For this review, take the finished solid that the model builds, in its own axes (mm). Give positions to 0.01 mm unless a question says otherwise; leave off trailing zeros. Write each loop counter-clockwise with the first axis right and the second up, starting at its lowest first coordinate (ties: lowest second). Pieces come first, ordered by that corner, then holes. Notation, with made-up numbers: (17.5, 65) -> (70.5, 65) arc R35 ccw to (70.5, 104) -> close; hole circle Ø2 at (-37, -40). An arc over 180 degrees is marked (long way). Answer as CSV lines item,"result".
```python
from build123d import *

# Parameters (mm, degrees)
BASPROSKE_W         = 6
BASPROSKE_H         = 9
TOOTHCUT_DEPTH      = 15.071247279
TEETHCUTS_COUNT     = 10
TEETHCUTS_ANGLE     = 324
BORSKE_R            = 2.5
BORE_DEPTH          = 50.0000508
BOSS_EXTRUDE2_DEPTH = 6


with BuildPart() as part:
    # BasProSke → Base-Revolve (revolve)
    with BuildSketch(Plane(origin=(0, 0, 0), x_dir=(1, 0, 0), z_dir=(0, 1, 0)), mode=Mode.PRIVATE) as base_revolve_sk:
        with Locations((3, 4.5)):
            Rectangle(BASPROSKE_W, BASPROSKE_H)
    revolve(base_revolve_sk.sketch.rotate(Axis((-10, 0, 0), (1, 0, 0)), 180), axis=Axis((-10, 0, 0), (1, 0, 0)))

    # TooCutSke → ToothCut (cut, through all)
    with BuildSketch(Plane(origin=(0, 0, 0), x_dir=(0, 0, -1), z_dir=(1, 0, 0))):
        with BuildLine():
            ThreePointArc((0.883878355, 5.554109745), (0, 5.624), (-0.883878355, 5.554109745))
            ThreePointArc((-0.883878355, 5.554109745), (-1.258245767, 7.379188248), (-2.637816971, 8.631324741))
            ThreePointArc((-2.637816971, 8.631324741), (0, 9.0254), (2.637816971, 8.631324741))
            ThreePointArc((2.637816971, 8.631324741), (1.258245767, 7.379188248), (0.883878355, 5.554109745))
        make_face()
    toothcut = extrude(amount=TOOTHCUT_DEPTH, mode=Mode.SUBTRACT)

    # TeethCuts: ToothCut ×10 about axis
    teethcuts_axis = Axis((-10, 0, 0), (1, 0, 0))
    for i in range(1, TEETHCUTS_COUNT):
        add(toothcut.rotate(teethcuts_axis, i * TEETHCUTS_ANGLE / (TEETHCUTS_COUNT - 1)), mode=Mode.SUBTRACT)

    # BorSke → Bore (cut, symmetric)
    with BuildSketch(Plane(origin=(0, 0, 0), x_dir=(0, 0, -1), z_dir=(1, 0, 0))):
        with Locations(Location((0, 0, 0), (0, 0, 180))):
            Circle(BORSKE_R)
    extrude(amount=BORE_DEPTH, both=True, mode=Mode.SUBTRACT)

    # Sketch1 → Boss-Extrude2 (add)
    with BuildSketch(Plane.ZY):
        with BuildLine():
            ThreePointArc((-3.953827157, 4.173517918), (-5.381277451, 5.377958207), (-7.24074087, 5.553133949))
            ThreePointArc((-7.24074087, 5.553133949), (-7.382280074, 5.363540427), (-7.518856208, 5.170341025))
            ThreePointArc((-7.518856208, 5.170341025), (-6.777648381, 3.456018504), (-5.191051196, 2.470625119))
            ThreePointArc((-5.191051196, 2.470625119), (-5.467623912, 1.776538701), (-5.651845645, 1.052445629))
            ThreePointArc((-5.651845645, 1.052445629), (-7.51462943, 1.18782406), (-9.121932655, 0.236579037))
            ThreePointArc((-9.121932655, 0.236579037), (-9.125, 0), (-9.121932655, -0.236579037))
            ThreePointArc((-9.121932655, -0.236579037), (-7.51462943, -1.18782406), (-5.651845645, -1.052445629))
            ThreePointArc((-5.651845645, -1.052445629), (-5.467623912, -1.776538701), (-5.191051196, -2.470625119))
            ThreePointArc((-5.191051196, -2.470625119), (-6.777648381, -3.456018504), (-7.518856208, -5.170341025))
            ThreePointArc((-7.518856208, -5.170341025), (-7.382280074, -5.363540427), (-7.24074087, -5.553133949))
            ThreePointArc((-7.24074087, -5.553133949), (-5.381277451, -5.377958207), (-3.953827157, -4.173517918))
            ThreePointArc((-3.953827157, -4.173517918), (-3.379177415, -4.651038701), (-2.747451628, -5.050001045))
            ThreePointArc((-2.747451628, -5.050001045), (-3.451836013, -6.779779466), (-3.043832247, -8.60236655))
            ThreePointArc((-3.043832247, -8.60236655), (-2.819780074, -8.678390711), (-2.593832177, -8.748580436))
            ThreePointArc((-2.593832177, -8.748580436), (-1.192460387, -7.513895108), (-0.74558108, -5.700448215))
            ThreePointArc((-0.74558108, -5.700448215), (0, -5.749), (0.74558108, -5.700448215))
            ThreePointArc((0.74558108, -5.700448215), (1.192460387, -7.513895108), (2.593832177, -8.748580436))
            ThreePointArc((2.593832177, -8.748580436), (2.819780074, -8.678390711), (3.043832247, -8.60236655))
            ThreePointArc((3.043832247, -8.60236655), (3.451836013, -6.779779466), (2.747451628, -5.050001045))
            ThreePointArc((2.747451628, -5.050001045), (3.379177415, -4.651038701), (3.953827157, -4.173517918))
            ThreePointArc((3.953827157, -4.173517918), (5.381277451, -5.377958207), (7.24074087, -5.553133949))
            ThreePointArc((7.24074087, -5.553133949), (7.382280074, -5.363540427), (7.518856208, -5.170341025))
            ThreePointArc((7.518856208, -5.170341025), (6.777648381, -3.456018504), (5.191051196, -2.470625119))
            ThreePointArc((5.191051196, -2.470625119), (5.467623912, -1.776538701), (5.651845645, -1.052445629))
            ThreePointArc((5.651845645, -1.052445629), (7.51462943, -1.18782406), (9.121932655, -0.236579037))
            ThreePointArc((9.121932655, -0.236579037), (9.125, 0), (9.121932655, 0.236579037))
            ThreePointArc((9.121932655, 0.236579037), (7.51462943, 1.18782406), (5.651845645, 1.052445629))
            ThreePointArc((5.651845645, 1.052445629), (5.467623912, 1.776538701), (5.191051196, 2.470625119))
            ThreePointArc((5.191051196, 2.470625119), (6.777648381, 3.456018504), (7.518856208, 5.170341025))
            ThreePointArc((7.518856208, 5.170341025), (7.382280074, 5.363540427), (7.24074087, 5.553133949))
            ThreePointArc((7.24074087, 5.553133949), (5.381277451, 5.377958207), (3.953827157, 4.173517918))
            ThreePointArc((3.953827157, 4.173517918), (3.379177415, 4.651038701), (2.747451628, 5.050001045))
            ThreePointArc((2.747451628, 5.050001045), (3.451836013, 6.779779466), (3.043832247, 8.60236655))
            ThreePointArc((3.043832247, 8.60236655), (2.819780074, 8.678390711), (2.593832177, 8.748580436))
            ThreePointArc((2.593832177, 8.748580436), (1.192460387, 7.513895108), (0.74558108, 5.700448215))
            ThreePointArc((0.74558108, 5.700448215), (0, 5.749), (-0.74558108, 5.700448215))
            ThreePointArc((-0.74558108, 5.700448215), (-1.192460387, 7.513895108), (-2.593832177, 8.748580436))
            ThreePointArc((-2.593832177, 8.748580436), (-2.819780074, 8.678390711), (-3.043832247, 8.60236655))
            ThreePointArc((-3.043832247, 8.60236655), (-3.451836013, 6.779779466), (-2.747451628, 5.050001045))
            ThreePointArc((-2.747451628, 5.050001045), (-3.379177415, 4.651038701), (-3.953827157, 4.173517918))
        make_face()
        with BuildLine():
            Line((-1.785357107, 1.45), (1.785357107, 1.45))
            ThreePointArc((1.785357107, 1.45), (0, -2.3), (-1.785357107, 1.45))
        make_face(mode=Mode.SUBTRACT)
    extrude(amount=-BOSS_EXTRUDE2_DEPTH)


solid = part.part
```
Q1. Draft analysis for pull direction Y (two halves, no side actions). For faces 1 (the flat face through (6, 2, 0)), 2 (the cylindrical face through (2.958, 4.645, 3.388)), state which applies: released by +Y, released by -Y, zero draft, split by the parting line, or undercut.
Answer block:
face 1,"zero draft"
face 2,"undercut"
Q2. Add section B-B (y = 0). Write out the cut boundary in (x, z) (3 decimals).
Answer block:
outline,"(0, -9.125) -> (6, -9.125) -> (6, -2.3) -> (0, -2.3) -> close; (0, 2.3) -> (6, 2.3) -> (6, 9.125) -> (0, 9.125) -> close"
Q3. Clearance check with flat-ended pins moving along their axes: pin 1 (1.8 mm diameter, centred on x = 3, z = 1, fed in from -Y); pin 2 (2 mm diameter, centred on x = 2.5, z = -5.5, fed in from -Y); pin 3 (1.5 mm diameter, centred on x = 4.5, y = -4, fed in from +Z). State where each tip first meets the part, or that it passes through.
Answer block:
pin 1,"stops at y = -8.32"
pin 2,"stops at y = -5.62"
pin 3,"stops at z = 7.45"
Q4. Add section C-C (y = -3). Write out the cut boundary in (x, z), plus the area to 3 significant figures.
Answer block:
outline,"(0, -6.29) -> (6, -6.29) -> (6, 6.29) -> (0, 6.29) -> close"
area,"75.5 mm2"
Q5. Add section A-A (z = 0). Write out the cut boundary in (x, y), plus the area to 3 significant figures.
Answer block:
outline,"(0, -5.75) -> (6, -5.75) -> (6, -2.3) -> (0, -2.3) -> close; (0, 1.45) -> (6, 1.45) -> (6, 5.75) -> (0, 5.75) -> close"
area,"46.5 mm2"
Q6. To check wall thickness, follow probe 1 along Y at (x, z) = (2.9, 0); probe 2 along Z at (x, y) = (3.35, 0) (3 decimals); probe 3 along Z at (x, y) = (5.75, 4.5). State the ranges of each line that lie inside material, in increasing order. Write a range as [from, to].
Answer block:
probe 1,"y = [-5.75, -2.3], [1.45, 5.75]"
probe 2,"z = [-9.125, -2.3], [2.3, 9.125]"
probe 3,"z = [-7.37, -4.19], [-3.58, 3.58], [4.19, 7.37]"
Q7. Add section D-D (z = 8). Write out the cut boundary in (x, y).
Answer block:
outline,"(0, -1.03) -> (6, -1.03) -> (6, 1.03) -> (0, 1.03) -> close"
